Could you check a few things on this drawing? It's one solid part, dimensions in mm from its lowest x, y, z. A direction names the side the tool comes from. Give positions to 0.01 mm unless a question says otherwise; leave off trailing zeros. Order: outer loops, then holes, each group sorted by start corner. A loop starts at its lowest first (then second) coordinate and runs counter-clockwise, first axis right, second up. Notation, with made-up numbers: M -1.75,-12 L 5.25,-12 A9 ccw 5.25,-3 Z; hole C 48,33.5 d8. An arc over 180 degrees is marked long. Use CSV: the item, a comma, the result in double quotes. Start each with the question number.
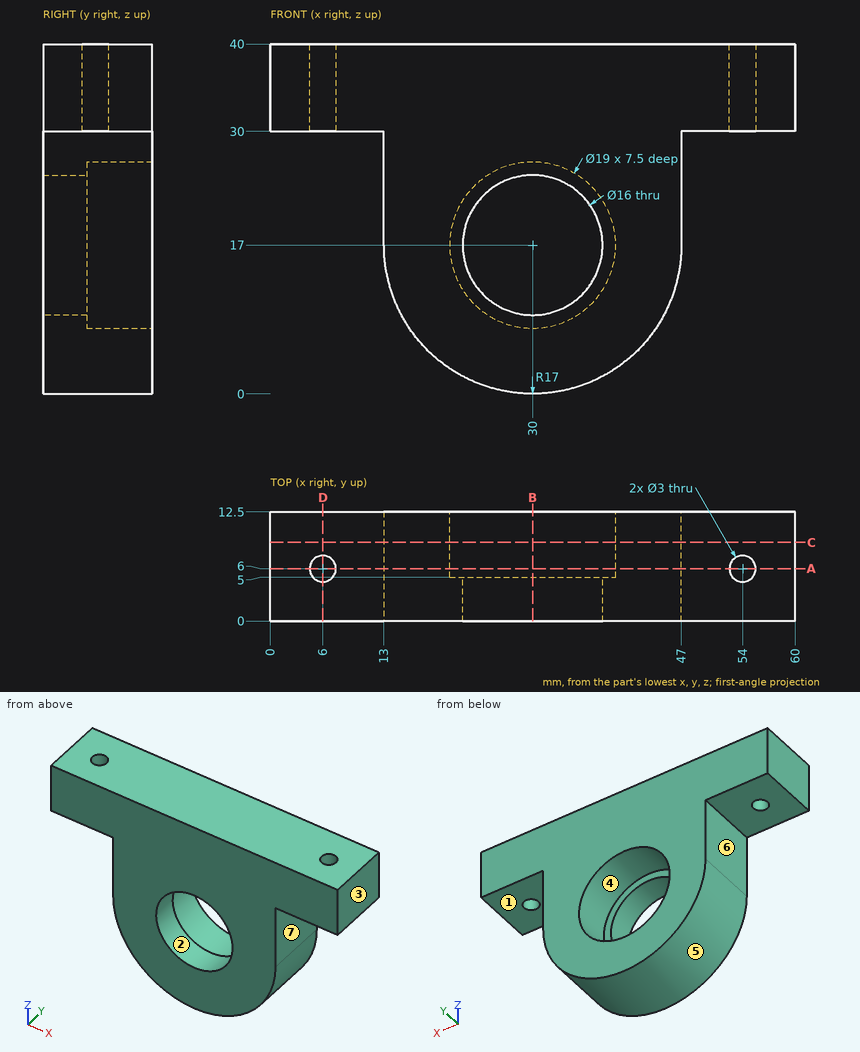
Q1. Imagine slicing it at A-A, the plane y = 6. Please give me the cut outline in (x, z).
Q2. Imagine slicing it at C-C, the plane y = 9. Please give me the cut outline in (x, z).
Q3. I need wall thicknesses on line 1 (X direction, y = 8.5, z = 16.5); line 2 (Y direction, x = 6, z = 36.75); line 3 (Z direction, x = 5.5, y = 3.5). Which ranges of each line are inside material? Lowest first, please. Write a range as [from, to].
Q4. We'd pull the mould along X, two halves only. Please class the marked faces 1, 2, 3 and 4: pulls with the +X half, pulls with the -X half, needs draft (parallel to the pull), parting line crosses it, or undercut.
Q5. Imagine slicing it at B-B, the plane x = 30. Please give me the cut outline in (y, z), then the cut area to 4 significant figures.
Q6. Imagine slicing it at D-D, the plane x = 6. Please give me the cut outline in (y, z), then the cut area to 3 significant figures.
Q7. For the marked faces 5, 6 and 7, which set-ups out of +Z, -Z, +X, -X, +Y, -Y let a thin tool reach every point of the face, with its end or its side?
Q8. For P1, Ø3, axis at x = 13.5, y = 6.5, coming from the -Z side; P2, Ø6, axis at x = 52, y = 4, coming from the -Z side; P3, Ø3, axis at y = 6.5, z = 27.5, coming from the -X side; P4, Ø5, axis at x = 6, y = 6, coming from the +Z side, each with a flat end and sliding along its axis, tell me the tip position at first contact or that it passes through.
Reply:
1,outline,"M 0,30 L 4.5,30 L 4.5,40 L 0,40 Z; M 7.5,30 L 13,30 L 13,17 A17 ccw 47,17 L 47,30 L 52.5,30 L 52.5,40 L 7.5,40 Z; M 55.5,30 L 60,30 L 60,40 L 55.5,40 Z; hole C 30,17 d19"
2,outline,"M 0,30 L 13,30 L 13,17 A17 ccw 47,17 L 47,30 L 60,30 L 60,40 L 0,40 Z; hole C 30,17 d19"
3,line 1,"x = [13.01, 20.51], [39.49, 46.99]"
3,line 2,"y = [0, 4.5], [7.5, 12.5]"
3,line 3,"z = [30, 40]"
4,face 1,"needs draft"
4,face 2,"undercut"
4,face 3,"pulls with the +X half"
4,face 4,"undercut"
5,outline,"M 0,0 L 12.5,0 L 12.5,7.5 L 5,7.5 L 5,9 L 0,9 Z; M 0,25 L 5,25 L 5,26.5 L 12.5,26.5 L 12.5,40 L 0,40 Z"
5,area,"277.5 mm^2"
6,outline,"M 0,30 L 4.5,30 L 4.5,40 L 0,40 Z; M 7.5,30 L 12.5,30 L 12.5,40 L 7.5,40 Z"
6,area,"95.0 mm^2"
7,face 5,"-Z, +Y, -Y"
7,face 6,"-Z, -X, +Y, -Y"
7,face 7,"-Z, +X, +Y, -Y"
8,P1,"stops at z = 9"
8,P2,"stops at z = 30"
8,P3,"stops at x = 13"
8,P4,"stops at z = 40"
